Here's the drawing with two shaded views (mm, measured from the low corner). I have some questions. Coordinates: 2 decimals unless noted, no trailing zeros. Order: outer loops, then holes, each group sorted by start corner. A loop starts at its lowest first (then second) coordinate and runs counter-clockwise, first axis right, second up. Notation, with made-up numbers: (87, 4) - (143, 4) arc R17 ccw to (143, 10) - close; hole circle Ø7 at (64, -30). An arc over 180 degrees is marked (long way). Answer as a JSON object with one key per item and string values. Group by question number.
(1) Imagine slicing it at D-D, the plane y = 50.5. Write out the boundary of the cut face in (x, z), and give its area (3 significant figures).
(2) Imagine slicing it at B-B, the plane y = 29. Write out the boundary of the cut face in (x, z), and give its area (3 significant figures).
(3) Please list where these lines run through material, in increasing order: probe 1 along Z at (x, y) = (7.75, 54.5); probe 2 along Z at (x, y) = (10.5, 30.5); probe 3 along X at (y, z) = (54.5, 45).
(4) We'd pull the mould along Z, two halves only. Please class the marked faces 1, 2 and 3: pulls with the +Z half, pulls with the -Z half, needs draft (parallel to the pull), parting line crosses it, or undercut.
(5) Imagine slicing it at C-C, the plane z = 45. Write out the boundary of the cut face in (x, y).
(6) Will these pins go through, and if not, where does the flat tip stop? P1, Ø3.5, axis at x = 7.5, z = 45, coming from the +Y side; P2, Ø19.5, axis at y = 35, z = 30, coming from the -X side; P3, Ø4, axis at x = 7, z = 27, coming from the +Y side.
(7) Imagine slicing it at A-A, the plane x = 7.5. Write out the boundary of the cut face in (y, z), and give its area (3 significant figures).
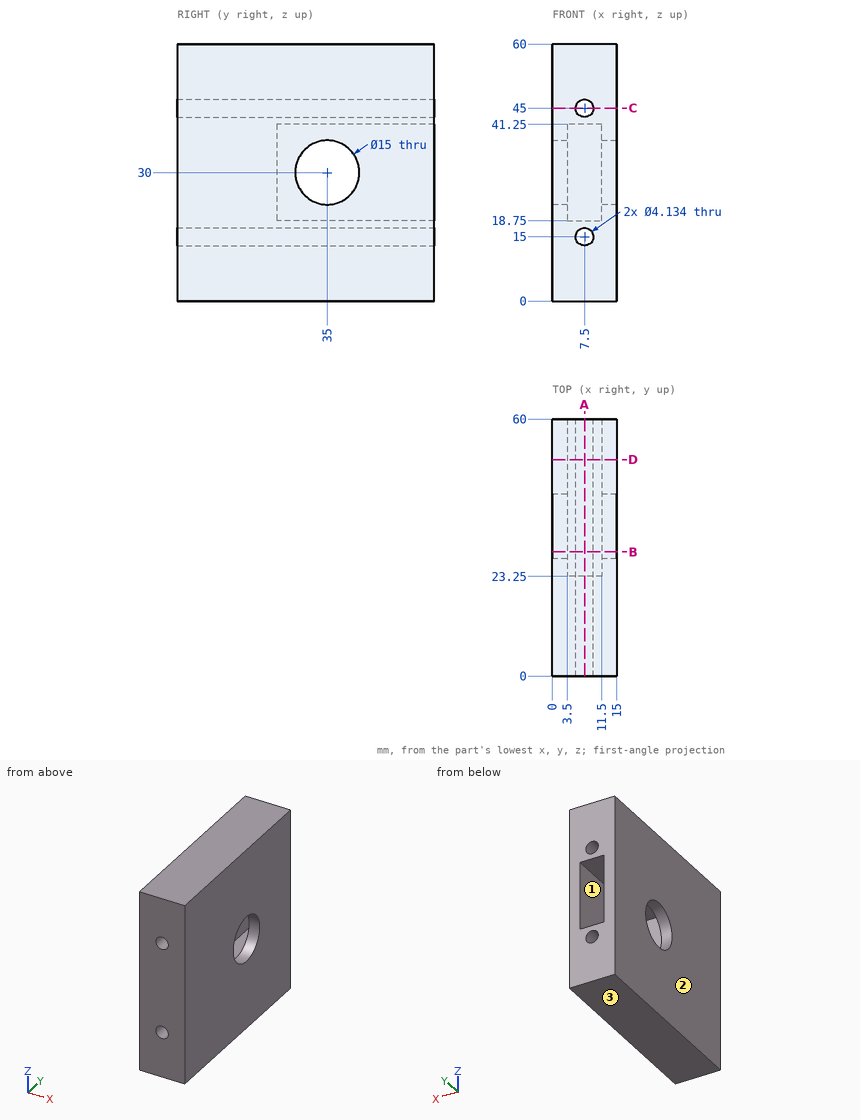
Result set:
{
 "1": {"outline": "(0, 0) - (15, 0) - (15, 60) - (0, 60) - close; hole (3.5, 18.75) - (11.5, 18.75) - (11.5, 41.25) - (3.5, 41.25) - close; hole circle Ø4.13 at (7.5, 15); hole circle Ø4.13 at (7.5, 45)", "area": "693 mm^2"},
 "2": {"outline": "(0, 0) - (15, 0) - (15, 25.5) - (11.5, 25.5) - (11.5, 18.75) - (3.5, 18.75) - (3.5, 25.5) - (0, 25.5) - close; (0, 34.5) - (3.5, 34.5) - (3.5, 41.25) - (11.5, 41.25) - (11.5, 34.5) - (15, 34.5) - (15, 60) - (0, 60) - close; hole circle Ø4.13 at (7.5, 15); hole circle Ø4.13 at (7.5, 45)", "area": "630 mm^2"},
 "3": {"probe 1": "z = 0 to 12.95, 17.05 to 18.75, 41.25 to 42.95, 47.05 to 60", "probe 2": "z = 0 to 18.75, 41.25 to 60", "probe 3": "x = 0 to 5.43, 9.57 to 15"},
 "4": {"face 1": "undercut", "face 2": "needs draft", "face 3": "pulls with the -Z half"},
 "5": {"outline": "(0, 0) - (5.43, 0) - (5.43, 60) - (0, 60) - close; (9.57, 0) - (15, 0) - (15, 60) - (9.57, 60) - close"},
 "6": {"P1": "passes through", "P2": "stops at x = 0", "P3": "stops at y = 23.25"},
 "7": {"outline": "(0, 0) - (60, 0) - (60, 12.93) - (0, 12.93) - close; (0, 17.07) - (60, 17.07) - (60, 18.75) - (23.25, 18.75) - (23.25, 41.25) - (60, 41.25) - (60, 42.93) - (0, 42.93) - close; (0, 47.07) - (60, 47.07) - (60, 60) - (0, 60) - close", "area": "2,280 mm^2"}
}
